Can you work these out from the drawing? Everything is in mm from the part's minimum corner. Give positions to 0.01 mm unless a question says otherwise; leave off trailing zeros. Order: outer loops, then holes, each group sorted by start corner. A loop starts at its lowest first (then second) coordinate and runs counter-clockwise, first axis right, second up. Notation, with made-up numbers: (-32, 26) - (-11, 26) arc R15 ccw to (-11, 40) - close; hole circle Ø9 at (-18, 64). An arc over 180 degrees is marked (long way). One line per question, with ' | ' between items.
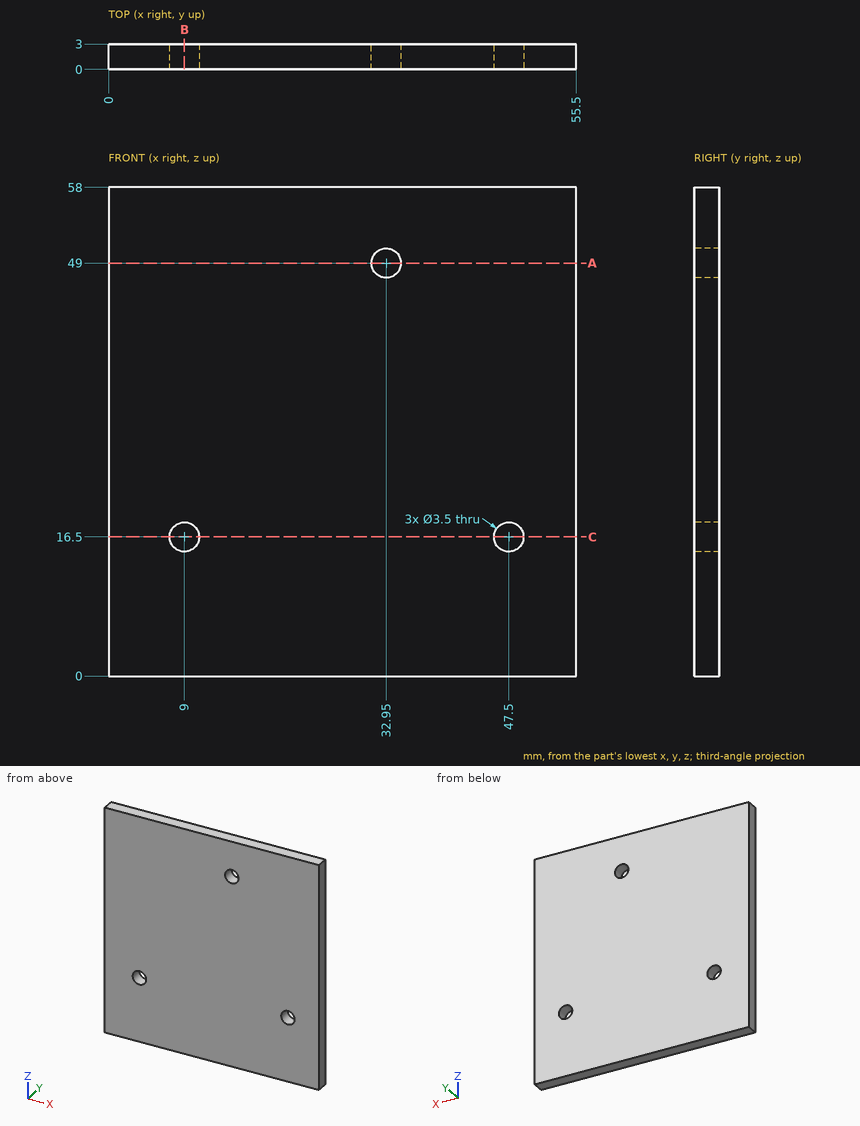
(1) Imagine slicing it at A-A (z = 49). List the corners of the cut face in (x, y) for me.
Answer below:
outline: (0, 0) - (31.2, 0) - (31.2, 3) - (0, 3) - close; (34.7, 0) - (55.5, 0) - (55.5, 3) - (34.7, 3) - close
(2) Imagine slicing it at C-C (z = 16.5). List the corners of the cut face in (x, y) for me.
Answer below:
outline: (0, 0) - (7.25, 0) - (7.25, 3) - (0, 3) - close; (10.75, 0) - (45.75, 0) - (45.75, 3) - (10.75, 3) - close; (49.25, 0) - (55.5, 0) - (55.5, 3) - (49.25, 3) - close
(3) If I drill on line 1 (Z direction, x = 47.5, y = 2.4); line 2 (X direction, y = 2.7, z = 47.5); line 3 (X direction, y = 1.55, z = 16), over which ranges is the centre line in solid material (lowest first)?
Answer below:
line 1: 0 to 14.75, 18.25 to 58 | line 2: 0 to 32.05, 33.85 to 55.5 | line 3: 0 to 7.32, 10.68 to 45.82, 49.18 to 55.5
(4) Imagine slicing it at B-B (x = 9). List the corners of the cut face in (y, z) for me, and give its area (4 significant figures).
Answer below:
outline: (0, 0) - (3, 0) - (3, 14.75) - (0, 14.75) - close; (0, 18.25) - (3, 18.25) - (3, 58) - (0, 58) - close | area: 163.5 mm^2
